Work out the finished part from the listing and answer in its coordinate system (mm). Face numbers are marked on the shaded views. Coordinates: 2 decimals unless noted, no trailing zeros. Order: outer loops, then holes, each group sorted by start corner. A loop starts at its lowest first (then second) coordinate and runs counter-clockwise, first axis right, second up.
1. The part is cut by section A-A, the plane x = -266. Give the vertices of the cut face in (y, z).
2. Find the intervals of material crossed by probe 1 along X at (y, z) = (-128, 1.4); probe 2 along Y at (x, z) = (-191, 1.95); probe 3 along Y at (x, z) = (-175, 0.35), in increasing order.
3. Flat-ended cylindrical pins translate along their axes: pin 1 Ø1 at (x, z) = (-208.5, 2) entering from -Y; pin 2 Ø1.5 at (x, z) = (-179, 1) entering from +Y. Find the tip coordinate at first contact, or state that the pin passes through.
4. Determine the mould class of the marked faces 1 and 2 for opening direction Z: +Z half, -Z half, draft (parallel to the pull), parting line (faces both ways), or undercut.
5. The part is cut by section C-C, the plane z = 2.15. Count the separate pieces of the cut face and the enclosed holes in it, then the cut area to 3 significant figures.
6. The part is cut by section B-B, the plane y = -50. Give the vertices of the cut face in (x, z), then the cut area to 3 significant figures.
```python
from build123d import *

# Parameters (mm, degrees)
BOSS_EXTRU_1_DEPTH = 3


with BuildPart() as part:
    # Esquisse1 → Boss.-Extru.1 (new body)
    with BuildSketch(Plane.XY):
        Polygon((-207.540430482, -98.290842938), (-228.119574859, -118.248029963), (-231.240854108, -118.563827288), (-272.565847516, -92.169507978), (-277.959789872, -89.716454796), (-284.165989399, -72.783703169), (-336.775785376, -57.698086926), (-338.147034057, -55.224288823), (-320.713145188, 5.574907028), (-318.239316427, 6.946262636), (-167.795259872, -36.183821192), (-156.425730461, -23.544541546), (-156.815310501, -19.508703235), (-167.175777529, -11.401531345), (-205.982988252, -11.401531345), (-221.327812729, -7.001473731), (-228.053301524, -5.072970852), (-324.305573392, 22.521130566), (-330.707501003, 18.97225141), (-353.72243999, -61.290379239), (-350.173829458, -67.692242105), (-294.328030452, -83.705767284), (-288.532091821, -99.519179156), (-251.042661762, -116.568594893), (-233.45174982, -134.735979634), (-226.135810249, -134.851076098), (-202.175390102, -111.650948678), (-133.415129641, -111.650948678), (-109.454709494, -134.851076098), (-102.138769923, -134.735979634), (-84.547857981, -116.568594893), (-47.058427922, -99.519179156), (-41.262489291, -83.705767284), (14.583309715, -67.692242105), (18.131920247, -61.290379239), (-4.88301874, 18.97225141), (-11.284946351, 22.521130566), (-107.537218219, -5.072970852), (-114.262707014, -7.001473731), (-123.876268292, -9.758118068), (-130.649820486, -22.415487094), (-129.8232917, -25.297935522), (-127.904950096, -24.747859919), (-17.351203316, 6.946262636), (-14.877374555, 5.574907028), (2.556514314, -55.224288823), (1.185265633, -57.698086926), (-51.424530344, -72.783703169), (-57.630729871, -89.716454796), (-63.024672228, -92.169507978), (-104.349665635, -118.563827288), (-107.470944884, -118.248029963), (-128.050089261, -98.290842938), (-133.151477342, -93.715936913), (-202.439042401, -93.715936913), align=None)
        Polygon((-214.696831686, -14.527657653), (-217.840116073, -13.876277124), (-219.975870353, -16.272750989), (-218.968340246, -19.320605385), (-215.825055858, -19.971985915), (-213.689301579, -17.575512049), align=None, mode=Mode.SUBTRACT)
        Polygon((-166.175746894, -24.833958909), (-169.385770719, -24.817214521), (-171.005283697, -27.588804506), (-169.414772849, -30.37713888), (-166.204749024, -30.393883267), (-164.585236046, -27.622293282), align=None, mode=Mode.SUBTRACT)
        Polygon((-115.672169645, -16.039488624), (-117.981174931, -13.809459943), (-121.066939064, -14.694102838), (-121.84369791, -17.808774414), (-119.534692623, -20.038803095), (-116.448928491, -19.154160201), align=None, mode=Mode.SUBTRACT)
        Polygon((-9.240055353, 15.320178943), (-12.039253575, 16.891491339), (-14.799649138, 15.252970767), (-14.76084648, 12.043137798), (-11.961648258, 10.471825402), (-9.201252694, 12.110345974), align=None, mode=Mode.SUBTRACT)
        Polygon((12.502351781, -60.574933915), (10.897318032, -57.794933915), (7.687250536, -57.794933915), (6.082216787, -60.574933915), (7.687250536, -63.354933915), (10.897318032, -63.354933915), align=None, mode=Mode.SUBTRACT)
        Polygon((-50.649763202, -94.526851626), (-51.178552765, -91.36063702), (-54.18496983, -90.235474912), (-56.662597331, -92.27652741), (-56.133807767, -95.442742016), (-53.127390703, -96.567904124), align=None, mode=Mode.SUBTRACT)
        Polygon((-104.440215275, -129.559925429), (-102.716844109, -126.851692582), (-104.200556971, -124.005092948), (-107.407640999, -123.866726161), (-109.131012166, -126.574959009), (-107.647299303, -129.421558643), align=None, mode=Mode.SUBTRACT)
        Polygon((-132.134816884, -105.032961295), (-129.102521286, -103.979530359), (-128.498671438, -100.826769871), (-130.927117189, -98.727440319), (-133.959412787, -99.780871255), (-134.563262635, -102.933631743), align=None, mode=Mode.SUBTRACT)
        Polygon((-200.986265397, -102.807259839), (-201.720052379, -99.68218544), (-204.793339689, -98.755126408), (-207.132840016, -100.953141775), (-206.399053033, -104.078216174), (-203.325765724, -105.005275206), align=None, mode=Mode.SUBTRACT)
        Polygon((-228.072581173, -129.499661036), (-226.456549288, -126.726039887), (-228.050559721, -123.939704646), (-231.260602039, -123.926990555), (-232.876633924, -126.700611704), (-231.282623491, -129.486946945), align=None, mode=Mode.SUBTRACT)
        Polygon((-279.761510176, -95.764600045), (-278.801584282, -92.701419409), (-280.974413583, -90.338508881), (-284.107168778, -91.03877899), (-285.067094671, -94.101959627), (-282.89426537, -96.464870154), align=None, mode=Mode.SUBTRACT)
        Polygon((-343.381773974, -63.412440235), (-341.674936445, -60.693756917), (-343.175966498, -57.856250598), (-346.38383408, -57.737427596), (-348.09067161, -60.456110913), (-346.589641557, -63.293617233), align=None, mode=Mode.SUBTRACT)
        Polygon((-323.377643582, 16.884689567), (-326.25776259, 15.467139628), (-326.470187835, 12.264108431), (-323.802494072, 10.478627174), (-320.922375064, 11.896177113), (-320.709949819, 15.09920831), align=None, mode=Mode.SUBTRACT)
    extrude(amount=BOSS_EXTRU_1_DEPTH)


solid = part.part
```
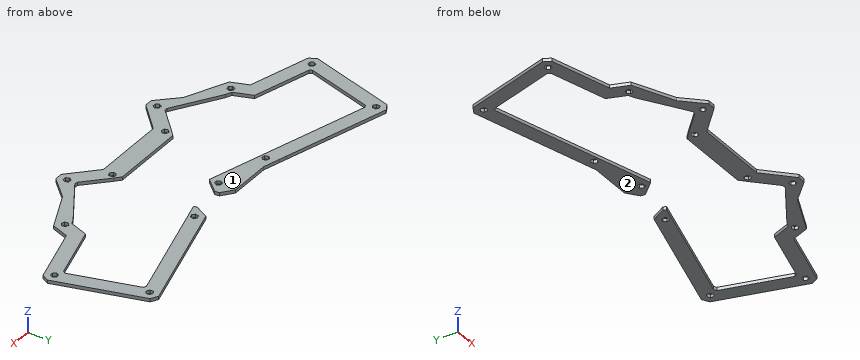
Geometry says:
1. outline: (-109.77, 0) - (-96.36, 0) - (-96.36, 3) - (-109.77, 3) - close; (-8.03, 0) - (5.81, 0) - (5.81, 3) - (-8.03, 3) - close
2. probe 1: x = -239.97 to -232.13, -227.2 to -219.06, -116.53 to -108.39, -103.45 to -95.62
2. probe 2: y = -111.65 to -93.72, -29.53 to -11.4
2. probe 3: y = -111.65 to -93.72, -34.12 to -11.4
3. pin 1: stops at y = -118.26
3. pin 2: stops at y = -11.4
4. face 1: +Z half
4. face 2: -Z half
5. separate pieces: 1
5. enclosed holes: 13
5. area: 11,700 mm2
6. outline: (-350.48, 0) - (-336.65, 0) - (-336.65, 3) - (-350.48, 3) - close; (1.06, 0) - (14.89, 0) - (14.89, 3) - (1.06, 3) - close
6. area: 83.0 mm2
